```python
from build123d import *

# Parameters (mm, degrees)
CROQUIS1_W              = 115
CROQUIS1_H              = 20.7
SALIENTE_EXTRUIR2_DEPTH = 3
CROQUIS6_R              = 1.5
CORTAR_EXTRUIR4_DEPTH   = 3
CROQUIS7_W              = 115
CROQUIS7_H              = 2
SALIENTE_EXTRUIR3_DEPTH = 9.7
CORTAR_EXTRUIR5_DEPTH   = 224


with BuildPart() as part:
    # Croquis1 → Saliente-Extruir2 (new body)
    with BuildSketch(Plane(origin=(0, 0, 0), x_dir=(1, 0, 0), z_dir=(0, 1, 0))):
        Rectangle(CROQUIS1_W, CROQUIS1_H)
    extrude(amount=SALIENTE_EXTRUIR2_DEPTH)

    # Croquis6 → Cortar-Extruir4 (cut)
    with BuildSketch(Plane(origin=(0, 3, 0), x_dir=(1, 0, 0), z_dir=(0, 1, 0))):
        with Locations((-42.5, 0)):
            Circle(CROQUIS6_R)
        Circle(CROQUIS6_R)
        with Locations((42.5, 0)):
            Circle(CROQUIS6_R)
    extrude(amount=-CORTAR_EXTRUIR4_DEPTH, mode=Mode.SUBTRACT)

    # Croquis7 → Saliente-Extruir3 (add)
    with BuildSketch(Plane(origin=(0, 3, 0), x_dir=(1, 0, 0), z_dir=(0, 1, 0))):
        with Locations((0, 9.35)):
            Rectangle(CROQUIS7_W, CROQUIS7_H)
        with Locations((0, -9.35)):
            Rectangle(CROQUIS7_W, CROQUIS7_H)
    extrude(amount=SALIENTE_EXTRUIR3_DEPTH)

    # Croquis9 → Cortar-Extruir5 (cut)
    with BuildSketch(Plane.ZY.offset(57.5)):
        Polygon((-10.35, 2.7), (-9.85, 2.7), (-10.35, 1.2), align=None)
        Polygon((10.35, 2.7), (9.85, 2.7), (10.35, 1.2), align=None)
    extrude(amount=-CORTAR_EXTRUIR5_DEPTH, mode=Mode.SUBTRACT)


solid = part.part
```
Design review of the part built by this model. Coordinates are the model's own, in mm. A direction names the side the tool comes from. Coordinates: 2 decimals unless noted, no trailing zeros. Order: outer loops, then holes, each group sorted by start corner. A loop starts at its lowest first (then second) coordinate and runs counter-clockwise, first axis right, second up.
1) Mouldability with a two-part tool opening along X and no side actions: class faces 1 (the flat face through (-1, 0, -2)), 2 (the flat face through (57.5, 2, 0)), 3 (the flat face through (-57.5, 2, 0)), 4 (the cylindrical face through (41, 2, 0)) as +X half, -X half, draft (parallel to the pull), parting line (faces both ways), or undercut.
2) Take a section at D-D, the plane z = 4.25. Give the boundary of the cut face in (x, y), and give its area (3 significant figures).
3) Take a section at A-A, the plane z = 0. Give the boundary of the cut face in (x, y), and give its area (3 significant figures).
4) Take a section at C-C, the plane x = 0. Give the boundary of the cut face in (y, z).
5) Clearance check with flat-ended pins moving along their axes: pin 1 (8 mm diameter, centred on x = -14, z = 3.5, fed in from -Y); pin 2 (4 mm diameter, centred on x = -35, z = 0, fed in from +Y); pin 3 (6 mm diameter, centred on y = 8.5, z = 0, fed in from +X). State where each tip first meets the part, or that it passes through.
6) For faces 5 (the flat face through (-1, 12.7, 9)), 6 (the flat face through (-1, 8, -8.35)), list the 3-axis set-ups (+Z, -Z, +X, -X, +Y, -Y) from which the entire face can be reached by the end or side of a thin tool; tool diameter is ignored.
7) Take a section at B-B, the plane y = 11.5. Give the boundary of the cut face in (x, z).
8) Wall thickness on line 1 along X through (y, z) = (0.8, 0); line 2 along Z through (x, y) = (20.5, 6); line 3 along Z through (x, y) = (0, 0.8): over which ranges is each line inside the solid? List them lowest first.
Returned:
1. face 1: draft
1. face 2: +X half
1. face 3: -X half
1. face 4: undercut
2. outline: (-57.5, 0) - (57.5, 0) - (57.5, 3) - (-57.5, 3) - close
2. area: 345 mm2
3. outline: (-57.5, 0) - (-44, 0) - (-44, 3) - (-57.5, 3) - close; (-41, 0) - (-1.5, 0) - (-1.5, 3) - (-41, 3) - close; (1.5, 0) - (41, 0) - (41, 3) - (1.5, 3) - close; (44, 0) - (57.5, 0) - (57.5, 3) - (44, 3) - close
3. area: 318 mm2
4. outline: (0, -10.35) - (1.2, -10.35) - (2.7, -9.85) - (2.7, -10.35) - (12.7, -10.35) - (12.7, -8.35) - (3, -8.35) - (3, -1.5) - (0, -1.5) - close; (0, 1.5) - (3, 1.5) - (3, 8.35) - (12.7, 8.35) - (12.7, 10.35) - (2.7, 10.35) - (2.7, 9.85) - (1.2, 10.35) - (0, 10.35) - close
5. pin 1: stops at y = 0
5. pin 2: stops at y = 3
5. pin 3: passes through
6. face 5: +Z, -Z, +X, -X, +Y
6. face 6: +X, -X, +Y
7. outline: (-57.5, -10.35) - (57.5, -10.35) - (57.5, -8.35) - (-57.5, -8.35) - close; (-57.5, 8.35) - (57.5, 8.35) - (57.5, 10.35) - (-57.5, 10.35) - close
8. line 1: x = -57.5 to -44, -41 to -1.5, 1.5 to 41, 44 to 57.5
8. line 2: z = -10.35 to -8.35, 8.35 to 10.35
8. line 3: z = -10.35 to -1.5, 1.5 to 10.35
